```python
from build123d import *

# Parameters (mm, degrees)
SKETCH1_W                 = 56
SKETCH1_H                 = 32
SKETCH1_W_2               = 52
SKETCH1_H_2               = 28
BOSS_EXTRUDE1_DEPTH       = 8
SKETCH2_W                 = 56
SKETCH2_H                 = 32
BOSS_EXTRUDE2_DEPTH       = 2
SKETCH3_R                 = 3.75
SKETCH3_R_2               = 1.75
SKETCH3_R_3               = 4.5
SKETCH3_R_4               = 2.5
BOSS_EXTRUDE3_DEPTH       = 6
MIRROR2_COPY_1_SKETCH_R   = 3.75
MIRROR2_COPY_1_SKETCH_R_2 = 1.75
MIRROR2_COPY_1_SKETCH_R_3 = 4.5
MIRROR2_COPY_1_SKETCH_R_4 = 2.5
MIRROR2_COPY_1_DEPTH      = 6
FILLET1_R                 = 1


with BuildPart() as part:
    # Sketch1 → Boss-Extrude1 (new body)
    with BuildSketch(Plane(origin=(0, 0, 0), x_dir=(1, 0, 0), z_dir=(0, 1, 0))):
        Rectangle(SKETCH1_W, SKETCH1_H)
        Rectangle(SKETCH1_W_2, SKETCH1_H_2, mode=Mode.SUBTRACT)
    extrude(amount=BOSS_EXTRUDE1_DEPTH)

    # Sketch2 → Boss-Extrude2 (add)
    with BuildSketch(Plane(origin=(0, 0, 0), x_dir=(1, 0, 0), z_dir=(0, 1, 0))):
        Rectangle(SKETCH2_W, SKETCH2_H)
    extrude(amount=BOSS_EXTRUDE2_DEPTH)

    # Sketch3 → Boss-Extrude3 (add)
    # profile 1 of 2: a face of its own
    with BuildSketch(Plane(origin=(0, 2, 0), x_dir=(1, 0, 0), z_dir=(0, 1, 0))):
        with Locations(Location((13.5, 0, 0), (0, 0, 270))):
            Circle(SKETCH3_R)
        with Locations(Location((13.5, 0, 0), (0, 0, 270))):
            Circle(SKETCH3_R_2, mode=Mode.SUBTRACT)
    # profile 2 of 2: a face of its own
    with BuildSketch(Plane(origin=(0, 2, 0), x_dir=(1, 0, 0), z_dir=(0, 1, 0))):
        with Locations(Location((20, 6.5, 0), (0, 0, 270))):
            Circle(SKETCH3_R_3)
        with Locations(Location((20, 6.5, 0), (0, 0, 270))):
            Circle(SKETCH3_R_4, mode=Mode.SUBTRACT)
    boss_extrude3 = extrude(amount=BOSS_EXTRUDE3_DEPTH)

    # Mirror1: Boss-Extrude3 across plane
    add(boss_extrude3.mirror(Plane.XY))

    # Mirror2: Boss-Extrude3 across plane
    add(boss_extrude3.mirror(Plane(origin=(0, 0, 0), x_dir=(0, 0, 1), z_dir=(1, 0, 0))))

    # Mirror2 copy 1 sketch → Mirror2 copy 1 (add)
    # profile 1 of 2: a face of its own
    with BuildSketch(Plane(origin=(0, 2, 0), x_dir=(-1, 0, 0), z_dir=(0, 1, 0))):
        with Locations(Location((13.5, 0, 0), (0, 0, 270))):
            Circle(MIRROR2_COPY_1_SKETCH_R)
        with Locations(Location((13.5, 0, 0), (0, 0, 270))):
            Circle(MIRROR2_COPY_1_SKETCH_R_2, mode=Mode.SUBTRACT)
    # profile 2 of 2: a face of its own
    with BuildSketch(Plane(origin=(0, 2, 0), x_dir=(-1, 0, 0), z_dir=(0, 1, 0))):
        with Locations(Location((20, 6.5, 0), (0, 0, 270))):
            Circle(MIRROR2_COPY_1_SKETCH_R_3)
        with Locations(Location((20, 6.5, 0), (0, 0, 270))):
            Circle(MIRROR2_COPY_1_SKETCH_R_4, mode=Mode.SUBTRACT)
    extrude(amount=MIRROR2_COPY_1_DEPTH)

    # Fillet1
    fillet1_edges = [part.edges().sort_by_distance(p)[0] for p in [
        (26, 5, 14),
        (26, 5, -14),
        (-26, 5, -14),
        (-26, 5, 14),
        (-28, 4, 16),
        (-28, 4, -16),
        (28, 4, -16),
        (28, 4, 16),
    ]]
    fillet(fillet1_edges, radius=FILLET1_R)


solid = part.part
```
Work out the finished part from the listing and answer in its coordinate system (mm). A direction names the side the tool comes from. Coordinates: 2 decimals unless noted, no trailing zeros. Loops run counter-clockwise (first coordinate to the right, second up) from the corner with the lowest first, then second, coordinate; pieces in that order, holes last. Notation, with made-up numbers: M -6.5,27.25 L 14.5,27.25 A16 ccw 14.5,38.25 Z; hole C -9.5,33 d10. An arc over 180 degrees is marked long. Use CSV: the item, a comma, the result in double quotes. Start each with the question number.
(1) Consider line 1 (X direction, y = 3.4, z = 6.5); line 2 (Z direction, x = -13.5, y = 4.5); line 3 (X direction, y = 4.1, z = 0). Determine where each line is inside the solid, lowest interval first.
(2) Find section C-C, the plane z = 6.5. Give the vertices of the cut face in (x, y), then the cut area to 3 significant figures.
(3) Find section A-A, the plane y = 6.25. State how many separate pieces and enclosed holes the cut face has, then the cut area to 3 significant figures.
(4) For faces 4 (the face through (-22, 5, 5)), 5 (the face through (18.1, 8, 4.6)), determine the directions among +Z, -Z, +X, -X, +Y, -Y from which every point of the face is accessible in a straight line to the end or side of a thin tool.
(5) Find section B-B, the plane x = 20. Give the vertices of the cut face in (y, z), then the cut area to 3 significant figures.
(6) For a pull along Z with two mould halves and no side action, classify faces 1 (the face through (22, 5, 5)), 2 (the face through (0, 0, 0)), 3 (the face through (25.699, 5.042, -13.715)) as +Z half, -Z half, draft (parallel to the pull), parting line (faces both ways), or undercut.
(7) Given pin 1 Ø6 at (x, z) = (20, -6.5) entering from +Y; pin 2 Ø1.5 at (x, z) = (-20.5, -1) entering from +Y, each flat-ended and moving along its own axis, determine where each tip first touches the part or whether it passes through.
(8) Find section D-D, the plane x = 5.5. Give the vertices of the cut face in (y, z).
Recorded:
1,line 1,"x = -28 to -26, -24.5 to -22.5, -17.5 to -15.5, 15.5 to 17.5, 22.5 to 24.5, 26 to 28"
1,line 2,"z = -16 to -14, -3.75 to -1.75, 1.75 to 3.75, 14 to 16"
1,line 3,"x = -28 to -26, -17.25 to -15.25, -11.75 to -9.75, 9.75 to 11.75, 15.25 to 17.25, 26 to 28"
2,outline,"M -28,0 L 28,0 L 28,8 L 26,8 L 26,2 L 24.5,2 L 24.5,8 L 22.5,8 L 22.5,2 L 17.5,2 L 17.5,8 L 15.5,8 L 15.5,2 L -15.5,2 L -15.5,8 L -17.5,8 L -17.5,2 L -22.5,2 L -22.5,8 L -24.5,8 L -24.5,2 L -26,2 L -26,8 L -28,8 Z"
2,area,"184 mm^2"
3,separate pieces,"7"
3,enclosed holes,"7"
3,area,"581 mm^2"
4,face 4,"+Y"
4,face 5,"+Z, -Z, +X, -X, +Y"
5,outline,"M 0,-16 L 8,-16 L 8,-14 L 2,-14 L 2,-11 L 8,-11 L 8,-9 L 2,-9 L 2,-4 L 8,-4 L 8,-2 L 2,-2 L 2,2 L 8,2 L 8,4 L 2,4 L 2,9 L 8,9 L 8,11 L 2,11 L 2,14 L 8,14 L 8,16 L 0,16 Z"
5,area,"136 mm^2"
6,face 1,"undercut"
6,face 2,"draft"
6,face 3,"undercut"
7,pin 1,"stops at y = 8"
7,pin 2,"stops at y = 2"
8,outline,"M 0,-16 L 8,-16 L 8,-14 L 2,-14 L 2,14 L 8,14 L 8,16 L 0,16 Z"
